Read the model definition and answer for the solid it produces. Units are mm, in the model's axes. A direction names the side the tool comes from. Round coordinates to 2 decimals unless told otherwise and drop trailing zeros. Order: outer loops, then holes, each group sorted by start corner. A loop starts at its lowest first (then second) coordinate and runs counter-clockwise, first axis right, second up. Notation, with made-up numbers: (10.25, 49) -> (39.25, 49) arc R23 ccw to (39.25, 70) -> close; hole circle Ø11 at (66, 15). An arc over 180 degrees is marked (long way). Use a Markdown table: item, result. Add a question column.
1. Consider L1, parallel to Z at x = -3.5, y = 4; L2, parallel to X at y = 12.75, z = 16; L3, parallel to Y at x = -0.5, z = 8. Determine where each line is inside the solid, lowest interval first. Write a range as [from, to].
2. The mould has two halves that part along Z. Classify faces 1 (the face through (26.346, 12.297, 16.521)), 2 (the face through (0, 8, 32)), 3 (the face through (-9.91, 6.42, 15.78)), 4 (the face through (-21.654, 12.297, 16.521)): +Z half, -Z half, draft (parallel to the pull), parting line (faces both ways), or undercut.
3. Section B-B, the plane y = 5 is taken. Give the vertices of the cut face in (x, z).
4. Section C-C, the plane z = 3 is taken. Give the vertices of the cut face in (x, y), then the cut area to 3 significant figures.
5. Given pin 1 (10 mm diameter, centred on x = 27.5, z = 8.5, fed in from -Y); pin 2 (1 mm diameter, centred on y = 9, z = 11, fed in from -X); pin 3 (3 mm diameter, centred on x = -12.5, z = 13, fed in from -Y), each flat-ended and moving along its own axis, determine where each tip first touches the part or whether it passes through.
6. For faces 5 (the face through (0.158, 4.601, 14.092)), 6 (the face through (-9, 9, 16)), 7 (the face through (9.882, 6.472, 15.776)), determine the directions among +Z, -Z, +X, -X, +Y, -Y from which every point of the face is accessible in a straight line to the end or side of a thin tool.
7. Section A-A, the plane x = -24 is taken. Give the vertices of the cut face in (y, z).
8. Section D-D, the plane x = 0.5 is taken. Give the vertices of the cut face in (y, z).
```python
from build123d import *

# Parameters (mm, degrees)
BOSS_EXTRUDE1_DEPTH                          = 32
SKETCH2_R                                    = 2
CUT_EXTRUDE1_DEPTH                           = 35.869794274
LPATTERN1_COUNT                              = 3
LPATTERN1_PITCH                              = 8
BOSS_EXTRUDE2_DEPTH                          = 9
BOSS_EXTRUDE2_DEPTH_BACK                     = 9
SKETCH3_W                                    = 32
SKETCH3_H                                    = 2
BOSS_EXTRUDE3_DEPTH                          = 35
BOSS_EXTRUDE3_DEPTH_BACK                     = 35
SKETCH4_W                                    = 32
SKETCH4_H                                    = 3
CSK_FOR_M4_COUNTERSUNK_FLAT_HEAD_SCR_2_COUNT = 2
CSK_FOR_M4_COUNTERSUNK_FLAT_HEAD_SCR_2_PITCH = 48


with BuildPart() as part:
    # Sketch1 → Boss-Extrude1 (new body)
    with BuildSketch(Plane.XY):
        Polygon((9, 0), (-9, 0), (-11.309401077, 4), (-9, 8), (9, 8), (11.309401077, 4), align=None)
    extrude(amount=BOSS_EXTRUDE1_DEPTH)

    # Sketch2 → Cut-Extrude1 (cut, symmetric)
    with BuildSketch(Plane(origin=(0, 0, 0), x_dir=(0, 0, -1), z_dir=(1, 0, 0))):
        with Locations((-24, 4)):
            Circle(SKETCH2_R)
    cut_extrude1 = extrude(amount=CUT_EXTRUDE1_DEPTH, both=True, mode=Mode.SUBTRACT)

    # LPattern1: Cut-Extrude1 ×3
    with Locations(*[(0, 0, -i * LPATTERN1_PITCH) for i in range(1, LPATTERN1_COUNT)]):
        add(cut_extrude1, mode=Mode.SUBTRACT)

    # Sketch3 → Boss-Extrude2 (add, two sides: drawn at the far end of the back side and taken through both)
    with BuildSketch(Plane(origin=(0, 0, 0), x_dir=(0, 0, -1), z_dir=(1, 0, 0)).offset(-BOSS_EXTRUDE2_DEPTH_BACK)):
        with Locations((-16, 9)):
            Rectangle(SKETCH3_W, SKETCH3_H)
    extrude(amount=BOSS_EXTRUDE2_DEPTH + BOSS_EXTRUDE2_DEPTH_BACK)

    # Sketch4 → Boss-Extrude3 (add, two sides: drawn at the far end of the back side and taken through both)
    with BuildSketch(Plane(origin=(0, 0, 0), x_dir=(0, 0, -1), z_dir=(1, 0, 0)).offset(-BOSS_EXTRUDE3_DEPTH_BACK)):
        with Locations((-16, 11.5)):
            Rectangle(SKETCH4_W, SKETCH4_H)
    extrude(amount=BOSS_EXTRUDE3_DEPTH + BOSS_EXTRUDE3_DEPTH_BACK)

    # Skizze3 → CSK for M4 Countersunk Flat Head Screw1 (revolve, cut)
    with BuildSketch(Plane(origin=(24, 10, 16), x_dir=(0, 0, -1), z_dir=(1, 0, 0))):
        Polygon((0, 0), (0, 3), (2.25, 3), (2.25, 2.45), (4.7, 0), align=None)
    csk_for_m4_countersunk_flat_head_screw1 = revolve(axis=Axis((24, 3.65, 16), (0, 1, 0)), mode=Mode.SUBTRACT)

    # CSK for M4 Countersunk Flat Head Scr 2: CSK for M4 Countersunk Flat Head Screw1 ×2
    with Locations(*[(-i * CSK_FOR_M4_COUNTERSUNK_FLAT_HEAD_SCR_2_PITCH, 0, 0) for i in range(1, CSK_FOR_M4_COUNTERSUNK_FLAT_HEAD_SCR_2_COUNT)]):
        add(csk_for_m4_countersunk_flat_head_screw1, mode=Mode.SUBTRACT)


solid = part.part
```
Verdict:
| question | item | result |
|---|---|---|
| 1 | L1 | z = [0, 6], [10, 14], [18, 22], [26, 32] |
| 1 | L2 | x = [-35, -26.25], [-21.75, 21.75], [26.25, 35] |
| 1 | L3 | y = [0, 2], [6, 13] |
| 2 | face 1 | undercut |
| 2 | face 2 | +Z half |
| 2 | face 3 | draft |
| 2 | face 4 | undercut |
| 3 | outline | (-10.73, 0) -> (10.73, 0) -> (10.73, 6.27) -> (-10.73, 6.27) -> close; (-10.73, 9.73) -> (10.73, 9.73) -> (10.73, 14.27) -> (-10.73, 14.27) -> close; (-10.73, 17.73) -> (10.73, 17.73) -> (10.73, 22.27) -> (-10.73, 22.27) -> close; (-10.73, 25.73) -> (10.73, 25.73) -> (10.73, 32) -> (-10.73, 32) -> close |
| 4 | outline | (-35, 10) -> (-9, 10) -> (-9, 8) -> (-11.31, 4) -> (-9, 0) -> (9, 0) -> (11.31, 4) -> (9, 8) -> (9, 10) -> (35, 10) -> (35, 13) -> (-35, 13) -> close |
| 4 | area | 408 mm2 |
| 5 | pin 1 | stops at y = 10 |
| 5 | pin 2 | stops at x = -9 |
| 5 | pin 3 | stops at y = 3.46 |
| 6 | face 5 | +X, -X |
| 6 | face 6 | +Z, -Z, -X |
| 6 | face 7 | +Z, -Z, +X |
| 7 | outline | (10, 0) -> (13, 0) -> (13, 13.75) -> (12.45, 13.75) -> (10, 11.3) -> close; (10, 20.7) -> (12.45, 18.25) -> (13, 18.25) -> (13, 32) -> (10, 32) -> close |
| 8 | outline | (0, 0) -> (13, 0) -> (13, 32) -> (0, 32) -> close; hole circle Ø4 at (4, 8); hole circle Ø4 at (4, 16); hole circle Ø4 at (4, 24) |
